Autodesk Inventor part; units mm, degrees
ref_plane "YZ Plane" through (0, 0, 0) normal (1, 0, 0) x (0, 1, 0)
ref_plane "XZ Plane" through (0, 0, 0) normal (0, 1, 0) x (-1, 0, 0)
ref_plane "XY Plane" through (0, 0, 0) normal (0, 0, 1) x (1, 0, 0)
sketch "Sketch1" plane through (0, 0, 0) normal (0, 1, 0) x (-1, 0, 0)
  line L0 (0, 0) -> (32, 0)
  arc A0 (32, -50) -> (32, 0) centre (32, -25) ccw
  line L1 (32, -50) -> (0, -50)
  dimension "d11" = 50
  dimension "d12" = 32
contour flange "Contour Flange1" sketch "Sketch1" thickness 4 bend radius 4 width 30 along (0, 1, 0) mid plane no both sides no wall seen from (-16, 0, 0) lies toward (0, 0, -1) curves L0 A0 L1
bend "Bend1"
corner "Corner1"
equation "\"d0\" = Thickness"
equation "\"d1\" = BendReliefWidth"
equation "\"d2\" = BendReliefDepth"
equation "\"d3\" = MinimumRemnant"
equation "\"d4\" = TransitionRadius"
equation "\"d6\" = BendRadius"
equation "\"d8\" = CornerReliefSize"
equation "\"d9\" = GapSize"
equation "\"d10\" = JacobiRadiusSize"
equation "\"BendRadius\" = Thickness"
equation "\"BendReliefWidth\" = Thickness"
equation "\"BendReliefDepth\" = 0.5 * Thickness"
equation "\"CornerReliefSize\" = 4 * Thickness"
equation "\"MinimumRemnant\" = 2 * Thickness"
equation "\"TransitionRadius\" = BendRadius"
equation "\"JacobiRadiusSize\" = BendRadius"
equation "\"GapSize\" = Thickness"
properties part number "bukket del" material "Steel"
The model under review builds one solid part; all positions refer to its coordinate system, in mm. A direction names the side the tool comes from. Coordinates: 2 decimals unless noted, no trailing zeros. Order: outer loops, then holes, each group sorted by start corner. A loop starts at its lowest first (then second) coordinate and runs counter-clockwise, first axis right, second up. Notation, with made-up numbers: (56.25, 25.5) -> (102.25, 25.5) arc R34 cw to (102.25, 56.5) -> close; hole circle Ø3 at (-27.5, 80). An arc over 180 degrees is marked (long way). Answer in a Markdown table with one row per item. Add a question column.
Item 1: Machinability: for faces 4 (the flat face through (-16, 15, -4)), 5 (the flat face through (-52, 30, -17)), which of the approach directions +Z, -Z, +X, -X, +Y, -Y give a long, thin tool a straight path to every point of the face, cutting with its end or side? Answer none if there is none.
Item 2: We need section B-B on y = 6.75. Write out the cut boundary in (x, z).
Item 3: We need section A-A on x = -18. Write out the cut boundary in (y, z), plus the area to 3 significant figures.
Item 4: We need section D-D on x = -49. Write out the cut boundary in (y, z).
Item 5: To check wall thickness, follow probe 1 along Z at (x, y) = (-27, 5); probe 2 along Z at (x, y) = (-36.5, 11.5); probe 3 along X at (y, z) = (16, -8). State the ranges of each line that lie inside material, in increasing order.
Item 6: We need section C-C on z = -25. Write out the cut boundary in (x, y).
Item 7: Clearance check with flat-ended pins moving along their axes: pin 1 (1 mm diameter, centred on y = 20.5, z = -39, fed in from +X); pin 2 (12 mm diameter, centred on x = -39.5, y = 9, fed in from -Z); pin 3 (3 mm diameter, centred on y = 11, z = -25.5, fed in from +X). State where each tip first meets the part, or that it passes through.
Item 8: Mouldability with a two-part tool opening along Z and no side actions: class faces 1 (the flat face through (0, 15, -2)), 2 (the flat face through (-16, 15, -50)), 3 (the flat face through (-16, 15, -46)) as +Z half, -Z half, draft (parallel to the pull), parting line (faces both ways), or undercut.
Final values:
| question | item | result |
|---|---|---|
| 1 | face 4 | +X, +Y, -Y |
| 1 | face 5 | +Z, -Z, +X, -X, +Y |
| 2 | outline | (-32, -50) -> (0, -50) -> (0, -46) -> (-32, -46) arc R21 cw to (-32, -4) -> (0, -4) -> (0, 0) -> (-32, 0) arc R25 ccw to start |
| 3 | outline | (0, -50) -> (30, -50) -> (30, -46) -> (0, -46) -> close; (0, -4) -> (30, -4) -> (30, 0) -> (0, 0) -> close |
| 3 | area | 240 mm2 |
| 4 | outline | (0, -43.33) -> (30, -43.33) -> (30, -37.33) -> (0, -37.33) -> close; (0, -12.67) -> (30, -12.67) -> (30, -6.67) -> (0, -6.67) -> close |
| 5 | probe 1 | z = -50 to -46, -4 to 0 |
| 5 | probe 2 | z = -49.59 to -45.51, -4.49 to -0.41 |
| 5 | probe 3 | x = -50.33 to -44.33 |
| 6 | outline | (-57, 0) -> (-53, 0) -> (-53, 30) -> (-57, 30) -> close |
| 7 | pin 1 | stops at x = -47.19 |
| 7 | pin 2 | stops at z = -49.95 |
| 7 | pin 3 | stops at x = -52.9 |
| 8 | face 1 | draft |
| 8 | face 2 | -Z half |
| 8 | face 3 | undercut |
